```python
from build123d import *

# Parameters (mm, degrees)
SKETCH1_W           = 15
SKETCH1_H           = 15
BOSS_EXTRUDE1_DEPTH = 11
FILLET1_R           = 2
BOSS_EXTRUDE2_DEPTH = 2.5


with BuildPart() as part:
    # Sketch1 → Boss-Extrude1 (new body)
    with BuildSketch(Plane.XY):
        Rectangle(SKETCH1_W, SKETCH1_H)
        with BuildLine():
            Line((-1.658312395, 2.5), (1.658312395, 2.5))
            ThreePointArc((1.658312395, 2.5), (0, -3), (-1.658312395, 2.5))
        make_face(mode=Mode.SUBTRACT)
    extrude(amount=-BOSS_EXTRUDE1_DEPTH)

    # Fillet1
    fillet1_edges = [part.edges().sort_by_distance(p)[0] for p in [
        (7.5, -7.5, -5.5),
        (-7.5, -7.5, -5.5),
        (-7.5, 7.5, -5.5),
        (7.5, 7.5, -5.5),
    ]]
    fillet(fillet1_edges, radius=FILLET1_R)

    # Sketch2 → Boss-Extrude2 (add)
    with BuildSketch(Plane.XY):
        with BuildLine():
            Line((7.5, -5.5), (7.5, 5.5))
            ThreePointArc((7.5, 5.5), (6.914213562, 6.914213562), (5.5, 7.5))
            Line((5.5, 7.5), (-5.5, 7.5))
            ThreePointArc((-5.5, 7.5), (-6.914213562, 6.914213562), (-7.5, 5.5))
            Line((-7.5, 5.5), (-7.5, -5.5))
            ThreePointArc((-7.5, -5.5), (-6.914213562, -6.914213562), (-5.5, -7.5))
            Line((-5.5, -7.5), (5.5, -7.5))
            ThreePointArc((5.5, -7.5), (6.914213562, -6.914213562), (7.5, -5.5))
        make_face()
    extrude(amount=BOSS_EXTRUDE2_DEPTH)


solid = part.part
```
Geometry: final body of the model. Coordinates: model frame, mm. A direction names the side the tool comes from. Coordinates: 2 decimals unless noted, no trailing zeros. Order: outer loops, then holes, each group sorted by start corner. A loop starts at its lowest first (then second) coordinate and runs counter-clockwise, first axis right, second up. Notation, with made-up numbers: (72.5, 10.5) -> (98.5, 10.5) arc R32 cw to (98.5, 44.5) -> close; hole circle Ø9 at (55, -30.75). An arc over 180 degrees is marked (long way). Write each question's results on one line, items separated by ' | '. Start each with the question number.
1) Material intervals for line 1 along Y through (x, z) = (0, -2.75); line 2 along X through (y, z) = (0, -5.5); line 3 along Z through (x, y) = (-0.75, -1.5), sorted ascending.
2) Cut plane B-B, the plane y = 0. Output: boundary loops of the cut face in (x, z), and give its area (4 significant figures).
3) Set-up query: faces 1 (the cylindrical face through (-6.9, 6.93, -4.34)), 2 (the flat face through (0, 0, 0)). Return all of +Z, -Z, +X, -X, +Y, -Y with unobstructed straight access to the full face (end or side cutting, diameter ignored); none if empty.
4) Cut plane C-C, the plane x = 0. Output: boundary loops of the cut face in (y, z), and give its area (3 significant figures).
5) Cut plane D-D, the plane x = 6.75. Output: boundary loops of the cut face in (y, z), and give its area (3 significant figures).
6) Mould query, pull axis X, two halves, no side actions, for faces 3 (the flat face through (-7.5, 0, -4)), 4 (the flat face through (0, 7.5, -4)), 5 (the cylindrical face through (0, -3, -5)). Classes: released by +X, released by -X, zero draft, split by the parting line, or undercut.
7) Cut plane A-A, the plane z = -8.25. Output: boundary loops of the cut face in (x, y), and give its area (3 significant figures).
Checks:
1) line 1: -7.5 to -3, 2.5 to 7.5 | line 2: -7.5 to -3, 3 to 7.5 | line 3: 0 to 2.5
2) outline: (-7.5, -11) -> (-3, -11) -> (-3, 0) -> (3, 0) -> (3, -11) -> (7.5, -11) -> (7.5, 2.5) -> (-7.5, 2.5) -> close | area: 136.5 mm^2
3) face 1: +Z, -Z, -X, +Y | face 2: -Z
4) outline: (-7.5, -11) -> (-3, -11) -> (-3, 0) -> (2.5, 0) -> (2.5, -11) -> (7.5, -11) -> (7.5, 2.5) -> (-7.5, 2.5) -> close | area: 142 mm^2
5) outline: (-7.06, -11) -> (7.06, -11) -> (7.06, 2.5) -> (-7.06, 2.5) -> close | area: 191 mm^2
6) face 3: released by -X | face 4: zero draft | face 5: undercut
7) outline: (-7.5, -5.5) arc R2 ccw to (-5.5, -7.5) -> (5.5, -7.5) arc R2 ccw to (7.5, -5.5) -> (7.5, 5.5) arc R2 ccw to (5.5, 7.5) -> (-5.5, 7.5) arc R2 ccw to (-7.5, 5.5) -> close; hole (-1.66, 2.5) arc R3 ccw (long way) to (1.66, 2.5) -> close | area: 194 mm^2
